```python
from build123d import *

# Parameters (mm, degrees)
SKETCH1_W           = 150
SKETCH1_H           = 72.26
BOSS_EXTRUDE1_DEPTH = 50
SKETCH2_R           = 3.6
CUT_EXTRUDE1_DEPTH  = 50
SKETCH3_W           = 30
SKETCH3_H           = 50
CUT_EXTRUDE2_DEPTH  = 18.75
CHAMFER1_SIZE       = 5
SKETCH4_W           = 80
SKETCH4_H           = 7.5
BOSS_EXTRUDE2_DEPTH = 7.5
CHAMFER2_SIZE       = 5
SKETCH5_W           = 150
SKETCH5_H           = 35
CUT_EXTRUDE3_DEPTH  = 68.26
SKETCH10_R          = 1.5
CUT_EXTRUDE4_DEPTH  = 4
SKETCH11_W          = 22
SKETCH11_H          = 3.75
CUT_EXTRUDE5_DEPTH  = 50
SKETCH13_W          = 80
SKETCH13_H          = 7.5
BOSS_EXTRUDE3_DEPTH = 7.5
SKETCH14_R          = 1.5
CUT_EXTRUDE6_DEPTH  = 7.5
CHAMFER3_SIZE       = 5
SKETCH19_W          = 20
SKETCH19_H          = 6.4
CUT_EXTRUDE10_DEPTH = 10
SKETCH20_W          = 14.825220809
SKETCH20_H          = 8.289370775
CUT_EXTRUDE11_DEPTH = 9
SKETCH21_W          = 20
SKETCH21_H          = 6.4
CUT_EXTRUDE12_DEPTH = 10


with BuildPart() as part:
    # Sketch1 → Boss-Extrude1 (new body)
    with BuildSketch(Plane(origin=(0, 0, 0), x_dir=(1, 0, 0), z_dir=(0, 1, 0))):
        Rectangle(SKETCH1_W, SKETCH1_H)
    extrude(amount=BOSS_EXTRUDE1_DEPTH)

    # Sketch2 → Cut-Extrude1 (cut)
    with BuildSketch(Plane(origin=(0, 50, 0), x_dir=(1, 0, 0), z_dir=(0, 1, 0))):
        with Locations(Location((-45, 0, 0), (0, 0, 270))):
            Circle(SKETCH2_R)
        with Locations(Location((45, 0, 0), (0, 0, 270))):
            Circle(SKETCH2_R)
    extrude(amount=-CUT_EXTRUDE1_DEPTH, mode=Mode.SUBTRACT)

    # Sketch3 → Cut-Extrude2 (cut)
    with BuildSketch(Plane(origin=(0, 0, -36.13), x_dir=(-1, 0, 0), z_dir=(0, 0, -1))):
        with Locations((60, 25)):
            Rectangle(SKETCH3_W, SKETCH3_H)
        with Locations((-60, 25)):
            Rectangle(SKETCH3_W, SKETCH3_H)
    extrude(amount=-CUT_EXTRUDE2_DEPTH, mode=Mode.SUBTRACT)

    # Chamfer1
    chamfer1_edges = [part.edges().sort_by_distance(p)[0] for p in [
        (-75, 25, -17.38),
        (-45, 25, -36.13),
        (75, 25, -17.38),
        (45, 25, -36.13),
    ]]
    chamfer(chamfer1_edges, length=CHAMFER1_SIZE)

    # Sketch4 → Boss-Extrude2 (add)
    with BuildSketch(Plane(origin=(0, 0, -36.13), x_dir=(-1, 0, 0), z_dir=(0, 0, -1))):
        with Locations((0, 46.25)):
            Rectangle(SKETCH4_W, SKETCH4_H)
    extrude(amount=BOSS_EXTRUDE2_DEPTH)

    # Chamfer2
    chamfer2_edges = [part.edges().sort_by_distance(p)[0] for p in [
        (40, 46.25, -43.63),
        (-40, 46.25, -43.63),
    ]]
    chamfer(chamfer2_edges, length=CHAMFER2_SIZE)

    # Sketch5 → Cut-Extrude3 (cut)
    with BuildSketch(Plane(origin=(0, 0, -36.13), x_dir=(-1, 0, 0), z_dir=(0, 0, -1))):
        with Locations((0, 25)):
            Rectangle(SKETCH5_W, SKETCH5_H)
    extrude(amount=-CUT_EXTRUDE3_DEPTH, mode=Mode.SUBTRACT)

    # Sketch10 → Cut-Extrude4 (cut)
    with BuildSketch(Plane.XY.offset(36.13)):
        with Locations((0, 26.25)):
            Circle(SKETCH10_R)
        with Locations((0, 18.75)):
            Circle(SKETCH10_R)
        with Locations((0, 11.25)):
            Circle(SKETCH10_R)
        with Locations((-7.5, 26.25)):
            Circle(SKETCH10_R)
        with Locations((-7.5, 18.75)):
            Circle(SKETCH10_R)
        with Locations((-7.5, 11.25)):
            Circle(SKETCH10_R)
        with Locations((7.5, 26.25)):
            Circle(SKETCH10_R)
        with Locations((7.5, 18.75)):
            Circle(SKETCH10_R)
        with Locations((7.5, 11.25)):
            Circle(SKETCH10_R)
    extrude(amount=-CUT_EXTRUDE4_DEPTH, mode=Mode.SUBTRACT)

    # Sketch11 → Cut-Extrude5 (cut)
    with BuildSketch(Plane(origin=(0, 50, 0), x_dir=(1, 0, 0), z_dir=(0, 1, 0))):
        with Locations((0, -30.255)):
            Rectangle(SKETCH11_W, SKETCH11_H)
    extrude(amount=-CUT_EXTRUDE5_DEPTH, mode=Mode.SUBTRACT)

    # Sketch13 → Boss-Extrude3 (add)
    with BuildSketch(Plane(origin=(0, 0, -36.13), x_dir=(-1, 0, 0), z_dir=(0, 0, -1))):
        with Locations((0, 3.75)):
            Rectangle(SKETCH13_W, SKETCH13_H)
    extrude(amount=BOSS_EXTRUDE3_DEPTH)

    # Sketch14 → Cut-Extrude6 (cut)
    with BuildSketch(Plane(origin=(0, 0, -43.63), x_dir=(-1, 0, 0), z_dir=(0, 0, -1))):
        with Locations((-15, 3.75)):
            Circle(SKETCH14_R)
        with Locations((15, 3.75)):
            Circle(SKETCH14_R)
    extrude(amount=-CUT_EXTRUDE6_DEPTH, mode=Mode.SUBTRACT)

    # Chamfer3
    chamfer3_edges = [part.edges().sort_by_distance(p)[0] for p in [
        (40, 3.75, -43.63),
        (-40, 3.75, -43.63),
    ]]
    chamfer(chamfer3_edges, length=CHAMFER3_SIZE)

    # Sketch19 → Cut-Extrude10 (cut)
    with BuildSketch(Plane(origin=(0, 50, 0), x_dir=(1, 0, 0), z_dir=(0, 1, 0))):
        with Locations((6.5, 0)):
            Rectangle(SKETCH19_W, SKETCH19_H)
    extrude(amount=-CUT_EXTRUDE10_DEPTH, mode=Mode.SUBTRACT)

    # Sketch20 → Cut-Extrude11 (cut)
    with BuildSketch(Plane.XY.offset(36.13)):
        with Locations((31.643078824, 22.688540842)):
            Rectangle(SKETCH20_W, SKETCH20_H)
    extrude(amount=-CUT_EXTRUDE11_DEPTH, mode=Mode.SUBTRACT)

    # Sketch21 → Cut-Extrude12 (cut)
    with BuildSketch(Plane.XZ):
        with Locations((-6.5, 0)):
            Rectangle(SKETCH21_W, SKETCH21_H)
    extrude(amount=-CUT_EXTRUDE12_DEPTH, mode=Mode.SUBTRACT)


solid = part.part
```
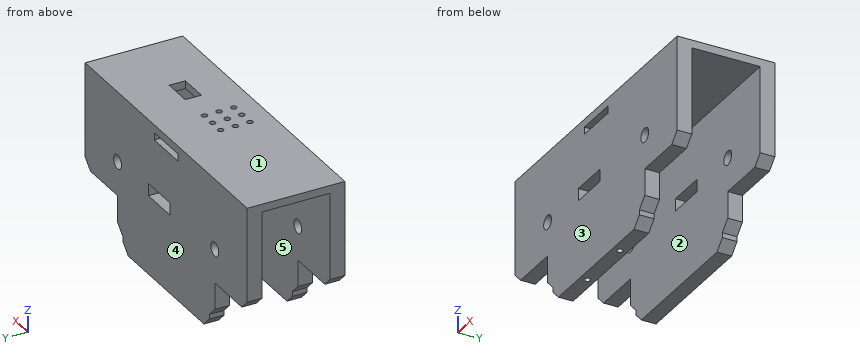
The model under review builds one solid part; all positions refer to its coordinate system, in mm. Face numbers are marked on the shaded views. A direction names the side the tool comes from. Round coordinates to 2 decimals unless told otherwise and drop trailing zeros. Loops run counter-clockwise (first coordinate to the right, second up) from the corner with the lowest first, then second, coordinate; pieces in that order, holes last.
Item 1: Take a section at D-D (y = 34). Write out the cut boundary in (x, z), then the cut area to 3 significant figures.
Determined:
outline: (-75, 32.13) - (75, 32.13) - (75, 36.13) - (-75, 36.13) - close
area: 600 mm2
Item 2: Take a section at B-B (x = 15). Write out the cut boundary in (y, z), then the cut area to 3 significant figures.
Determined:
outline: (0, -43.63) - (2.25, -43.63) - (2.25, -36.13) - (5.25, -36.13) - (5.25, -43.63) - (7.5, -43.63) - (7.5, 32.13) - (42.5, 32.13) - (42.5, 3.2) - (50, 3.2) - (50, 36.13) - (0, 36.13) - close; (42.5, -43.63) - (50, -43.63) - (50, -3.2) - (42.5, -3.2) - close
area: 1,270 mm2
Item 3: Clearance check with flat-ended pins moving along their axes: pin 1 Ø2.5 at (x, y) = (0, 26.25) entering from +Z; pin 2 Ø5 at (x, y) = (-7.5, 18.75) entering from -Z; pin 3 Ø4 at (x, y) = (62.5, 4.5) entering from -Z; pin 4 Ø6 at (y, z) = (2.5, -26.5) entering from +X. State where each tip first meets the part, or that it passes through.
Determined:
pin 1: passes through
pin 2: stops at z = 32.13
pin 3: stops at z = -17.38
pin 4: stops at x = 45
Item 4: Take a section at C-C (x = 0). Give the number of separate pieces and of enclosed holes in the cut face, then the cut area to 3 significant figures.
Determined:
separate pieces: 8
enclosed holes: 0
area: 1,150 mm2
Item 5: Take a section at A-A (z = -33). Write out the cut boundary in (x, y), then the cut area to 3 significant figures.
Determined:
outline: (-43.13, 0) - (43.13, 0) - (43.13, 7.5) - (-43.13, 7.5) - close; (-43.13, 42.5) - (43.13, 42.5) - (43.13, 50) - (-43.13, 50) - close
area: 1,290 mm2
Item 6: Mouldability with a two-part tool opening along Y and no side actions: class the marked faces 3, 4 and 5 as released by +Y, released by -Y, zero draft, split by the parting line, or undercut.
Determined:
face 3: released by -Y
face 4: released by +Y
face 5: undercut
Item 7: For line 1 (Z direction, x = 8.5, y = 48); line 2 (X direction, y = 48, z = 0); line 3 (Y direction, x = -15, z = -38.25), list the stretches that pass through material, from the lowest coordinate up.
Determined:
line 1: z = -43.63 to -3.2, 3.2 to 28.38, 32.13 to 36.13
line 2: x = -75 to -48.6, -41.4 to -3.5, 16.5 to 41.4, 48.6 to 75
line 3: y = 0 to 2.25, 5.25 to 7.5, 42.5 to 50
Item 8: For the marked faces 1 and 2, list the 3-axis set-ups (+Z, -Z, +X, -X, +Y, -Y) from which the entire face can be reached by the end or side of a thin tool; tool diameter is ignored.
Determined:
face 1: +Z, +X, -X, +Y, -Y
face 2: -Z, +X, -X
